The listing builds one solid part. Answer for the finished solid, in the listing's coordinates (mm). Face numbers are marked on the shaded views. A direction names the side the tool comes from. Round coordinates to 2 decimals unless told otherwise and drop trailing zeros. Loops run counter-clockwise (first coordinate to the right, second up) from the corner with the lowest first, then second, coordinate; pieces in that order, holes last. Notation, with made-up numbers: (77.25, 81) -> (85.25, 81) arc R27 ccw to (85.25, 106) -> close; hole circle Ø9 at (-14, -4). An arc over 180 degrees is marked (long way). Write each question's results on one line, items separated by ' | '. Start each with the question number.
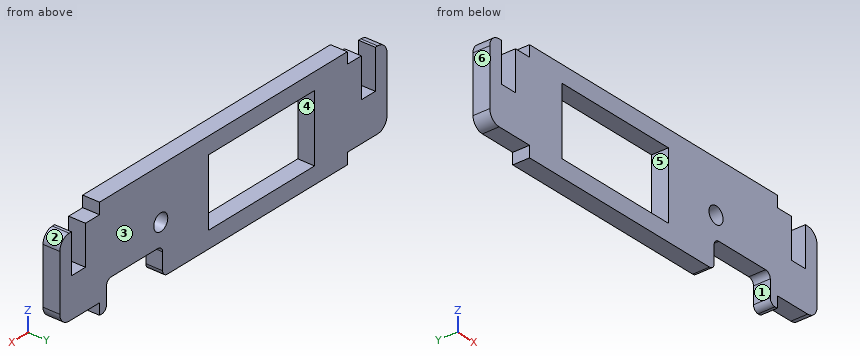
from build123d import *

# Parameters (mm, degrees)
BOSS_EXTRUDE1_DEPTH = 3
SKETCH2_W           = 22.7
SKETCH2_H           = 12
CUT_EXTRUDE1_DEPTH  = 3
SKETCH3_W           = 3
SKETCH3_H           = 7
CUT_EXTRUDE2_DEPTH  = 3
SKETCH4_R           = 1.5
CUT_EXTRUDE3_DEPTH  = 3


with BuildPart() as part:
    # Sketch1 → Boss-Extrude1 (new body)
    with BuildSketch(Plane(origin=(0, 0, 0), x_dir=(1, 0, 0), z_dir=(0, 1, 0))):
        with BuildLine():
            Line((-9.820632273, 11.009972833), (-9.820632273, 1.009972833))
            ThreePointArc((-9.820632273, 1.009972833), (-10.40641871, -0.404240729), (-11.820632273, -0.990027167))
            Line((-11.820632273, -0.990027167), (-18.320632273, -0.990027167))
            Line((-18.320632273, -0.990027167), (-18.320632273, -2.990027167))
            Line((-18.320632273, -2.990027167), (-71.320632273, -2.990027167))
            Line((-71.320632273, -2.990027167), (-71.320632273, -0.990027167))
            Line((-71.320632273, -0.990027167), (-77.820632273, -0.990027167))
            ThreePointArc((-77.820632273, -0.990027167), (-79.234845835, -0.404240729), (-79.820632273, 1.009972833))
            Line((-79.820632273, 1.009972833), (-79.820632273, 11.009972833))
            ThreePointArc((-79.820632273, 11.009972833), (-79.234845835, 12.424186396), (-77.820632273, 13.009972833))
            Line((-77.820632273, 13.009972833), (-71.320632273, 13.009972833))
            Line((-71.320632273, 13.009972833), (-71.320632273, 15.009972833))
            Line((-71.320632273, 15.009972833), (-32.820632273, 15.009972833))
            ThreePointArc((-32.820632273, 15.009972833), (-32.113525492, 14.717079615), (-31.820632273, 14.009972833))
            Line((-31.820632273, 14.009972833), (-31.820632273, 11.009972833))
            ThreePointArc((-31.820632273, 11.009972833), (-31.527739054, 10.302866052), (-30.820632273, 10.009972833))
            Line((-30.820632273, 10.009972833), (-20.820632273, 10.009972833))
            ThreePointArc((-20.820632273, 10.009972833), (-20.113525492, 10.302866052), (-19.820632273, 11.009972833))
            Line((-19.820632273, 11.009972833), (-19.820632273, 14.009972833))
            ThreePointArc((-19.820632273, 14.009972833), (-19.527739054, 14.717079615), (-18.820632273, 15.009972833))
            Line((-18.820632273, 15.009972833), (-18.320632273, 15.009972833))
            Line((-18.320632273, 15.009972833), (-18.320632273, 13.009972833))
            Line((-18.320632273, 13.009972833), (-11.820632273, 13.009972833))
            ThreePointArc((-11.820632273, 13.009972833), (-10.40641871, 12.424186396), (-9.820632273, 11.009972833))
        make_face()
    extrude(amount=BOSS_EXTRUDE1_DEPTH)

    # Sketch2 → Cut-Extrude1 (cut)
    with BuildSketch(Plane(origin=(0, 3, 0), x_dir=(1, 0, 0), z_dir=(0, 1, 0))):
        with Locations((-52.970632273, 6.009972833)):
            Rectangle(SKETCH2_W, SKETCH2_H)
    extrude(amount=-CUT_EXTRUDE1_DEPTH, mode=Mode.SUBTRACT)

    # Sketch3 → Cut-Extrude2 (cut)
    with BuildSketch(Plane(origin=(0, 3, 0), x_dir=(1, 0, 0), z_dir=(0, 1, 0))):
        with Locations((-13.820632273, 2.509972833)):
            Rectangle(SKETCH3_W, SKETCH3_H)
        with Locations((-75.820632273, 2.509972833)):
            Rectangle(SKETCH3_W, SKETCH3_H)
    extrude(amount=-CUT_EXTRUDE2_DEPTH, mode=Mode.SUBTRACT)

    # Sketch4 → Cut-Extrude3 (cut)
    with BuildSketch(Plane(origin=(0, 3, 0), x_dir=(1, 0, 0), z_dir=(0, 1, 0))):
        with Locations(Location((-31.420632273, 6.109972833, 0), (0, 0, 270))):
            Circle(SKETCH4_R)
    extrude(amount=-CUT_EXTRUDE3_DEPTH, mode=Mode.SUBTRACT)


solid = part.part
Item 1: Determine the mould class of the marked faces 1, 2, 3 and 4 for opening direction X: +X half, -X half, draft (parallel to the pull), parting line (faces both ways), or undercut.
Item 2: The part is cut by section C-C, the plane z = -2.75. Give the vertices of the cut face in (x, y), plus the area to 3 significant figures.
Item 3: Each of these flat-tipped pins is pushed along its axis until it touches: pin 1 Ø1.5 at (y, z) = (2, -12) entering from -X; pin 2 Ø0.9 at (x, y) = (-73, 2) entering from +Z; pin 3 Ø1.5 at (x, y) = (-75.5, 1) entering from -Z. Where does it stop, or does it pass through?
Item 4: For the marked faces 5 and 6, determine the directions among +Z, -Z, +X, -X, +Y, -Y from which every point of the face is accessible in a straight line to the end or side of a thin tool.
Item 5: Straight lines are drawn through the part: L1, parallel to X at y = 2.55, z = -1.25; L2, parallel to X at y = 2.95, z = -11.25; L3, parallel to Z at x = -61, y = 2.45. For each, find the intervals that lie inside material, in ascending order. Write a range as [from, to].
Item 6: The part is cut by section B-B, the plane x = -49. Give the vertices of the cut face in (y, z).
Item 7: The part is cut by section D-D, the plane y = 1.6. Give the number of separate pieces and of enclosed holes in the cut face, plus the area to 3 significant figures.
Item 8: The part is cut by section A-A, the plane z = -8.75. Give the vertices of the cut face in (x, y), plus the area to 3 significant figures.
Report:
1) face 1: undercut | face 2: +X half | face 3: draft | face 4: undercut
2) outline: (-79.82, 0) -> (-77.32, 0) -> (-77.32, 3) -> (-79.82, 3) -> close; (-74.32, 0) -> (-64.32, 0) -> (-64.32, 3) -> (-74.32, 3) -> close; (-41.62, 0) -> (-15.32, 0) -> (-15.32, 3) -> (-41.62, 3) -> close; (-12.32, 0) -> (-9.82, 0) -> (-9.82, 3) -> (-12.32, 3) -> close | area: 124 mm2
3) pin 1: stops at x = -79.81 | pin 2: stops at z = 0.99 | pin 3: stops at z = -13.01
4) face 5: +Y, -Y | face 6: +Z, -Z, -X, +Y, -Y
5) L1: x = [-79.82, -77.32], [-74.32, -64.32], [-41.62, -15.32], [-12.32, -9.82] | L2: x = [-79.81, -64.32], [-41.62, -31.82], [-19.82, -9.84] | L3: z = [-15.01, -12.01], [-0.01, 2.99]
6) outline: (0, -15.01) -> (3, -15.01) -> (3, -12.01) -> (0, -12.01) -> close; (0, -0.01) -> (3, -0.01) -> (3, 2.99) -> (0, 2.99) -> close
7) separate pieces: 1 | enclosed holes: 2 | area: 807 mm2
8) outline: (-79.82, 0) -> (-64.32, 0) -> (-64.32, 3) -> (-79.82, 3) -> close; (-41.62, 0) -> (-9.82, 0) -> (-9.82, 3) -> (-41.62, 3) -> close | area: 142 mm2
